Geometry: see drawing. Coordinates: mm, zero at the bounding-box minimum. Coordinates: 2 decimals unless noted, no trailing zeros. Write each loop counter-clockwise with the first axis right and the second up, starting at its lowest first coordinate (ties: lowest second). Pieces come first, ordered by that corner, then holes. Notation, with made-up numbers: (41, 85.5) - (89, 85.5) arc R28 ccw to (89, 108.5) - close; hole circle Ø1 at (-12, -3.5). An arc over 180 degrees is marked (long way). Use CSV: the item, a comma, the result in double quotes.
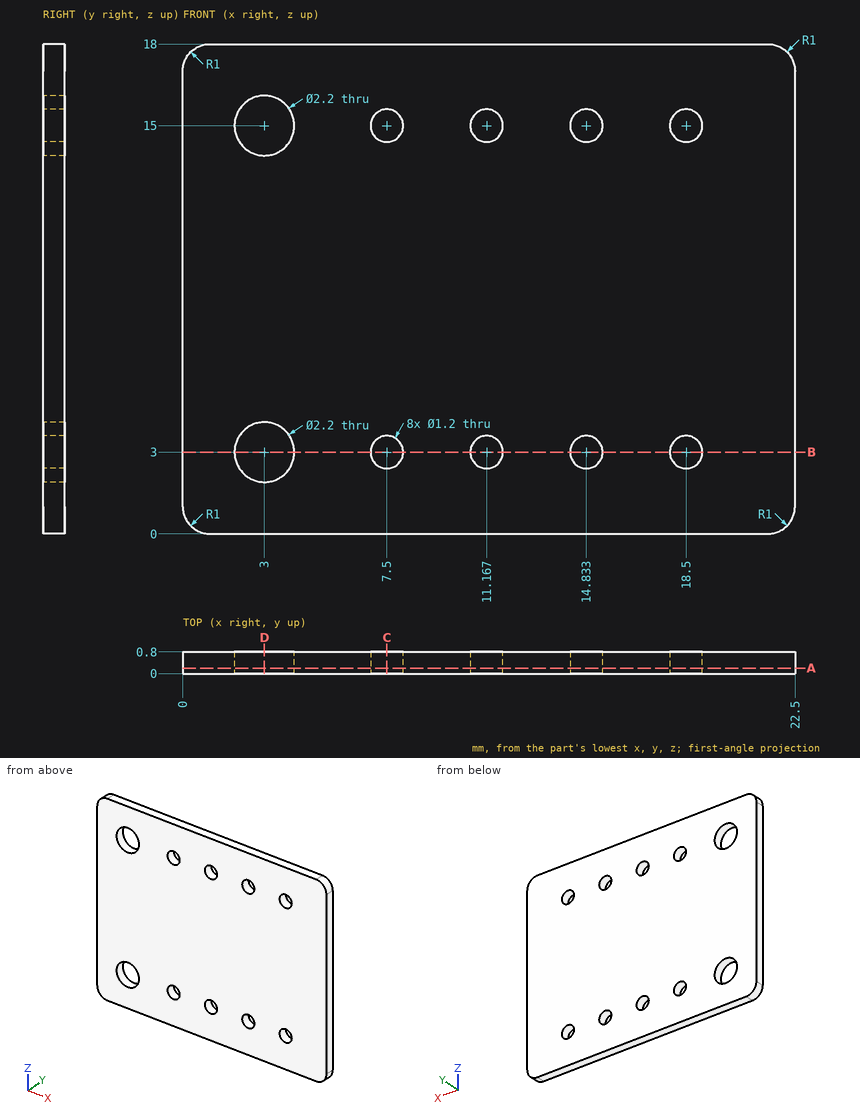
(1) Cut plane A-A on y = 0.2. State how many separate pieces and enclosed holes the cut face has.
Check values:
separate pieces,"1"
enclosed holes,"10"
(2) Ray query, probe 1 along Z at (x, y) = (3, 0.65); probe 2 along Z at (x, y) = (2, 0.65) (1 decimal); probe 3 along X at (y, z) = (0.75, 15.5) (1 decimal). Return the intervals inside material, ascending. Write a range as from..to.
Check values:
probe 1,"0..1.9, 4.1..13.9, 16.1..18"
probe 2,"0..2.5, 3.5..14.5, 15.5..18"
probe 3,"0..2, 4..7.2, 7.8..10.8, 11.5..14.5, 15.2..18.2, 18.8..22.5"
(3) Pin query (flat end, axial travel): pin 1 Ø0.7 at (x, z) = (14.83, 15) entering from +Y. Return the tip coordinate at first contact, or that it passes through.
Check values:
pin 1,"through"
(4) Cut plane D-D on x = 3. Return loops of the section in (y, z).
Check values:
outline,"(0, 0) - (0.8, 0) - (0.8, 1.9) - (0, 1.9) - close; (0, 4.1) - (0.8, 4.1) - (0.8, 13.9) - (0, 13.9) - close; (0, 16.1) - (0.8, 16.1) - (0.8, 18) - (0, 18) - close"
(5) Cut plane B-B on z = 3. Return loops of the section in (x, y).
Check values:
outline,"(0, 0) - (1.9, 0) - (1.9, 0.8) - (0, 0.8) - close; (4.1, 0) - (6.9, 0) - (6.9, 0.8) - (4.1, 0.8) - close; (8.1, 0) - (10.57, 0) - (10.57, 0.8) - (8.1, 0.8) - close; (11.77, 0) - (14.23, 0) - (14.23, 0.8) - (11.77, 0.8) - close; (15.43, 0) - (17.9, 0) - (17.9, 0.8) - (15.43, 0.8) - close; (19.1, 0) - (22.5, 0) - (22.5, 0.8) - (19.1, 0.8) - close"
(6) Cut plane C-C on x = 7.5. Return loops of the section in (y, z), and give its area (3 significant figures).
Check values:
outline,"(0, 0) - (0.8, 0) - (0.8, 2.4) - (0, 2.4) - close; (0, 3.6) - (0.8, 3.6) - (0.8, 14.4) - (0, 14.4) - close; (0, 15.6) - (0.8, 15.6) - (0.8, 18) - (0, 18) - close"
area,"12.5 mm^2"
